For this review, take the finished solid that the model builds, in its own axes (mm). Give positions to 0.01 mm unless a question says otherwise; leave off trailing zeros. Write each loop counter-clockwise with the first axis right and the second up, starting at its lowest first coordinate (ties: lowest second). Pieces come first, ordered by that corner, then holes. Notation, with made-up numbers: M 49.5,-24.5 L 83.5,-24.5 A21 ccw 83.5,13.5 Z; hole C 5,30.5 d6. An arc over 180 degrees is marked long. Use one line per item in the form item = value. Start each with the question number.
Q1. Consider section A-A on x = 28. Write out the cut boundary in (y, z) (3 decimals).
Q2. Consider section C-C on z = 2.15. Give the number of separate pieces and of enclosed holes in the cut face, and give its area (3 significant figures).
Q3. Consider section B-B on x = 268. Write out the cut boundary in (y, z) (3 decimals), and give its area (4 significant figures).
Q4. For probe 1 along Y at (x, z) = (75, 0.75) (3 decimals); probe 2 along Y at (x, z) = (225, 0.7) (3 decimals); probe 3 along X at (y, z) = (-15, 0.8), list the stretches that pass through material, from the lowest coordinate up. Write a range as [from, to].
Q5. Mouldability with a two-part tool opening along Z and no side actions: class faces 1 (the flat face through (147, 0, 3)), 2 (the flat face through (147, 0, 0)) as released by +Z, released by -Z, zero draft, split by the parting line, or undercut.
```python
from build123d import *

# Parameters (mm, degrees)
SKETCH_1_W          = 450
SKETCH_1_H          = 45.25
EXTRUDE_1_DEPTH     = 3
SKETCH_1_3_W        = 21.6
SKETCH_1_3_H        = 27.1
SKETCH_1_3_W_2      = 45.25
SKETCH_1_3_H_2      = 26
CUT_EXTRUDE_2_DEPTH = 3
SKETCH_2_R          = 2.15
CUT_EXTRUDE_3_DEPTH = 5
SKETCH_3_R          = 2.15
CUT_EXTRUDE_4_DEPTH = 5


with BuildPart() as part:
    # 草圖1 → 填料-伸長1 (new body)
    with BuildSketch(Plane.XY):
        with Locations((150, 0)):
            Rectangle(SKETCH_1_W, SKETCH_1_H)
    extrude(amount=EXTRUDE_1_DEPTH)

    # 草圖1<3> → 除料-伸長2 (cut)
    with BuildSketch(Plane.XY):
        with Locations((-37.4, 0)):
            Rectangle(SKETCH_1_3_W, SKETCH_1_3_H)
        with Locations((174.2, 0)):
            Rectangle(SKETCH_1_3_W_2, SKETCH_1_3_H_2)
        with Locations((24.2, 0)):
            Rectangle(SKETCH_1_3_W_2, SKETCH_1_3_H_2)
        with Locations((112.6, 0)):
            Rectangle(SKETCH_1_3_W, SKETCH_1_3_H)
        with Locations((324.2, 0)):
            Rectangle(SKETCH_1_3_W_2, SKETCH_1_3_H_2)
        with Locations((262.6, 0)):
            Rectangle(SKETCH_1_3_W, SKETCH_1_3_H)
    extrude(amount=CUT_EXTRUDE_2_DEPTH, mode=Mode.SUBTRACT)

    # 草圖2 → 除料-伸長3 (cut)
    with BuildSketch(Plane(origin=(0, 0, 0), x_dir=(-1, 0, 0), z_dir=(0, 0, -1))):
        with Locations((-359.3, 14.725)):
            Circle(SKETCH_2_R)
        with Locations((-359.3, -14.725)):
            Circle(SKETCH_2_R)
        with Locations((59.3, 14.725)):
            Circle(SKETCH_2_R)
        with Locations((59.3, -14.725)):
            Circle(SKETCH_2_R)
    extrude(amount=-CUT_EXTRUDE_3_DEPTH, mode=Mode.SUBTRACT)

    # 草圖3 → 除料-伸長4 (cut)
    with BuildSketch(Plane(origin=(0, 0, 0), x_dir=(-1, 0, 0), z_dir=(0, 0, -1))):
        with Locations((-225.014075293, 6.925)):
            Circle(SKETCH_3_R)
        with Locations((-225, -6.925)):
            Circle(SKETCH_3_R)
        with Locations((-75.000000001, 6.925)):
            Circle(SKETCH_3_R)
        with Locations((-75, -8.025)):
            Circle(SKETCH_3_R)
    extrude(amount=-CUT_EXTRUDE_4_DEPTH, mode=Mode.SUBTRACT)


solid = part.part
```
Working result:
q1.outline = M -22.625,0 L -13,0 L -13,3 L -22.625,3 Z; M 13,0 L 22.625,0 L 22.625,3 L 13,3 Z
q2.separate_pieces = 1
q2.enclosed_holes = 14
q2.area = 15,000 mm²
q3.outline = M -22.625,0 L -13.55,0 L -13.55,3 L -22.625,3 Z; M 13.55,0 L 22.625,0 L 22.625,3 L 13.55,3 Z
q3.area = 54.45 mm²
q4.probe_1 = [-22.625, -10.175], [-5.875, 4.775], [9.075, 22.625]
q4.probe_2 = [-22.625, -9.075], [-4.775, 4.775], [9.075, 22.625]
q4.probe_3 = [-75, -61.43], [-57.17, 357.17], [361.43, 375]
q5.face_1 = released by +Z
q5.face_2 = released by -Z
